Input: dimensioned drawing with shaded views. Units: mm. Origin: part minimum x, y, z. A direction names the side the tool comes from. Round coordinates to 2 decimals unless told otherwise and drop trailing zeros. Loops run counter-clockwise (first coordinate to the right, second up) from the corner with the lowest first, then second, coordinate; pieces in that order, holes last. Notation, with made-up numbers: M -6.75,33.25 L 41.25,33.25 A28 ccw 41.25,53.25 Z; hole C 28.25,9.5 d7. An arc over 180 degrees is marked long. One line per item, written item: value.
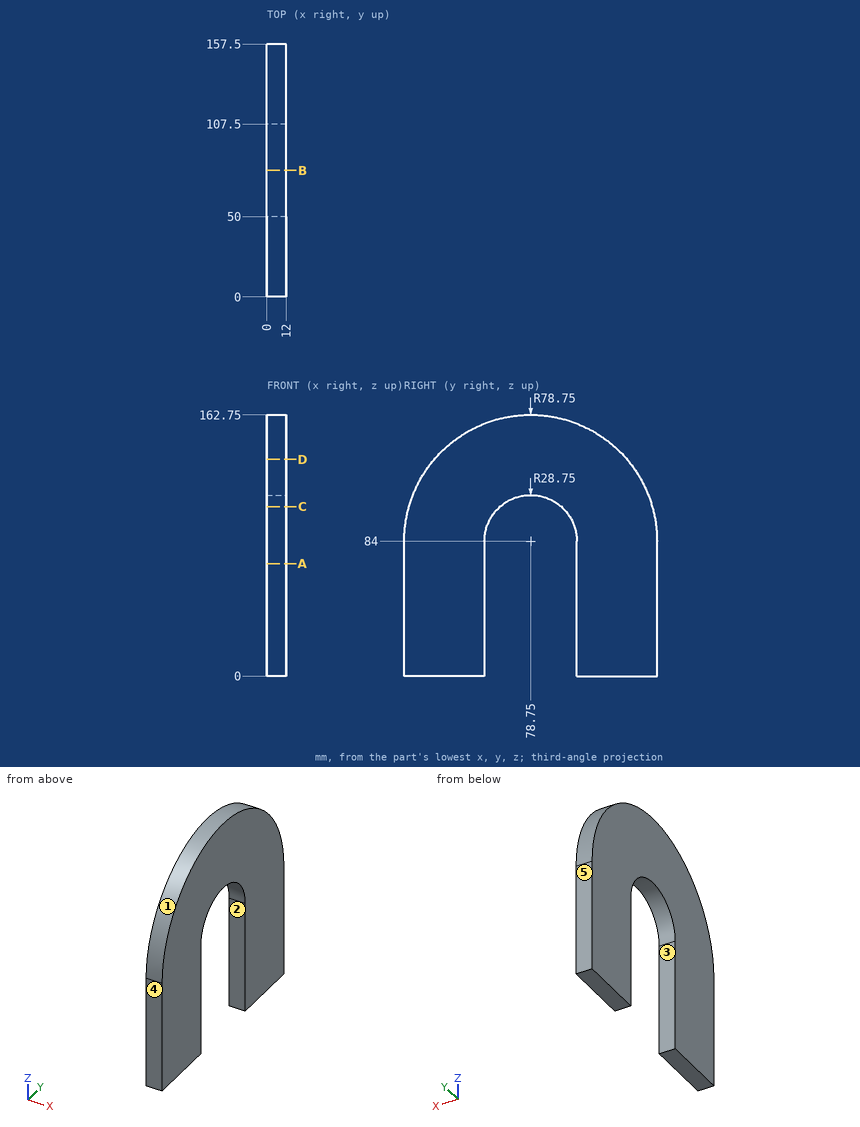
1. Section query C-C (z = 105.5). Return the cut outline in (x, y).
Report:
outline: M 0,2.99 L 12,2.99 L 12,59.66 L 0,59.66 Z; M 0,97.84 L 12,97.84 L 12,154.51 L 0,154.51 Z
2. Ray query, line 1 (Y direction, x = 1.5, z = 48.5); line 2 (Y direction, x = 2.5, z = 93) (3 decimals); line 3 (Z direction, x = 2.5, y = 133). Return the intervals inside material, ascending. Write a range as [from, to].
Report:
line 1: y = [0, 50], [107.5, 157.5]
line 2: y = [0.516, 51.445], [106.055, 156.984]
line 3: z = [0, 141.08]
3. Pull-direction query (Y, two-part tool) for the marked faces 3, 4 and 5; classes: released by +Y, released by -Y, zero draft, split by the parting line, or undercut.
Report:
face 3: undercut
face 4: released by -Y
face 5: released by +Y
4. Section query A-A (z = 70). Return the cut outline in (x, y), and give its area (3 significant figures).
Report:
outline: M 0,0 L 12,0 L 12,50 L 0,50 Z; M 0,107.5 L 12,107.5 L 12,157.5 L 0,157.5 Z
area: 1,200 mm2
5. Pin query (flat end, axial travel): pin 1 (1 mm diameter, centred on x = 7, y = 98.5, fed in from -Z); pin 2 (1 mm diameter, centred on y = 129, z = 72, fed in from -X); pin 3 (6 mm diameter, centred on x = 9, z = 97, fed in from +Y); pin 4 (4 mm diameter, centred on x = 11, z = 110, fed in from +Y). Return the tip coordinate at first contact, or that it passes through.
Report:
pin 1: stops at z = 104.41
pin 2: stops at x = 0
pin 3: stops at y = 156.86
pin 4: stops at y = 153.75
6. Section query B-B (y = 78.75). Return the cut outline in (x, z).
Report:
outline: M 0,112.75 L 12,112.75 L 12,162.75 L 0,162.75 Z
7. Section query D-D (z = 135). Return the cut outline in (x, y), and give its area (3 significant figures).
Report:
outline: M 0,18.75 L 12,18.75 L 12,138.75 L 0,138.75 Z
area: 1,440 mm2
8. Reachability of the marked faces 1 and 2 from +Z, -Z, +X, -X, +Y, -Y: full face, straight path, thin tool, end or side. Return the list, or none.
Report:
face 1: +Z, +X, -X
face 2: -Z, +X, -X
